Could you check a few things on this model? Use its own coordinates, in mm. Face numbers are marked on the shaded views. A direction names the side the tool comes from. Give positions to 0.01 mm unless a question says otherwise; leave off trailing zeros. Order: outer loops, then holes, each group sorted by start corner. A loop starts at its lowest first (then second) coordinate and runs counter-clockwise, first axis right, second up. Notation, with made-up numbers: (45, 33) -> (86, 33) arc R19 ccw to (86, 58) -> close; hole circle Ø11 at (14.25, 73.25). An arc over 180 degrees is marked (long way). Write each question's results on one line, items separated by ' | '.
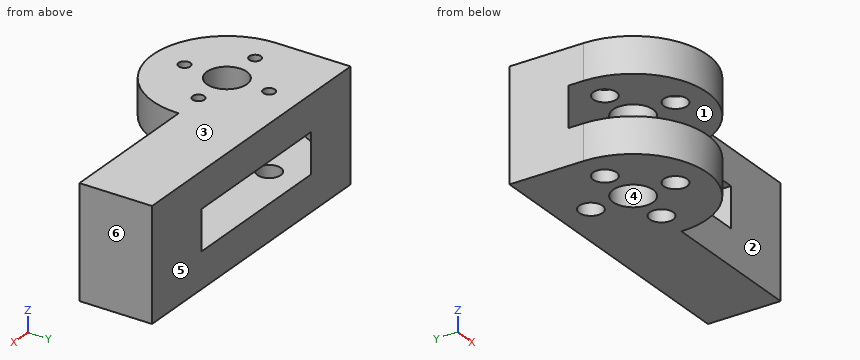
```python
from build123d import *

# Parameters (mm, degrees)
SKETCH1_R           = 3.429
BOSS_EXTRUDE1_DEPTH = 9.525
CUT_EXTRUDE1_START  = -9.525
CUT_EXTRUDE1_DEPTH  = 3.429
SKETCH4_R           = 1.004000024
CUT_EXTRUDE2_DEPTH  = 20.05
SKETCH5_R           = 2.000000064
CUT_EXTRUDE3_DEPTH  = 14.954


with BuildPart() as part:
    # Sketch1 → Boss-Extrude1 (new body, symmetric)
    with BuildSketch(Plane.XY):
        with BuildLine():
            Line((-12.7, 0), (-12.7, 12.7))
            Line((-12.7, 12.7), (38.1, 12.7))
            Line((38.1, 12.7), (38.1, 0.254))
            Line((38.1, 0.254), (12.697459746, 0.254))
            ThreePointArc((12.697459746, 0.254), (0.127006351, -12.699364921), (-12.7, 0))
        make_face()
        Circle(SKETCH1_R, mode=Mode.SUBTRACT)
    extrude(amount=BOSS_EXTRUDE1_DEPTH, both=True)

    # Sketch3 → Cut-Extrude1 (cut, symmetric)
    with BuildSketch(Plane.XY.offset(9.525).offset(CUT_EXTRUDE1_START)):
        with BuildLine():
            Line((25.4, 12.7), (25.4, 0.254))
            Line((25.4, 0.254), (12.951509565, 0.254))
            ThreePointArc((12.951509565, 0.254), (-9.069614104, -9.24922786), (0, 12.954))
            Line((0, 12.954), (0, 12.7))
            Line((0, 12.7), (25.4, 12.7))
        make_face()
    extrude(amount=CUT_EXTRUDE1_DEPTH, both=True, mode=Mode.SUBTRACT)

    # Sketch4 → Cut-Extrude2 (cut, through all)
    with BuildSketch(Plane.XY.offset(9.525)):
        with Locations((7.249999978, 0)):
            Circle(SKETCH4_R)
        with Locations((0, -7.249999978)):
            Circle(SKETCH4_R)
        with Locations((-7.249999978, 0)):
            Circle(SKETCH4_R)
        with Locations((0, 7.249999978)):
            Circle(SKETCH4_R)
    extrude(amount=-CUT_EXTRUDE2_DEPTH, mode=Mode.SUBTRACT)

    # Sketch5 → Cut-Extrude3 (cut)
    with BuildSketch(Plane(origin=(0, 0, -9.525), x_dir=(-1, 0, 0), z_dir=(0, 0, -1))):
        with Locations((7.249999978, 0)):
            Circle(SKETCH5_R)
        with Locations((0, -7.249999978)):
            Circle(SKETCH5_R)
        with Locations((-7.249999978, 0)):
            Circle(SKETCH5_R)
        with Locations((0, 7.249999978)):
            Circle(SKETCH5_R)
    extrude(amount=-CUT_EXTRUDE3_DEPTH, mode=Mode.SUBTRACT)


solid = part.part
```
Q1. Suppose I cut it at D-D on y = 7.25. Please give me the cut outline in (x, z) (3 decimals).
Here are the results:
outline: (-12.7, -9.525) -> (-2, -9.525) -> (-2, -3.429) -> (-10.735, -3.429) -> (-10.735, 3.429) -> (-2, 3.429) -> (-2, 5.429) -> (-1.004, 5.429) -> (-1.004, 9.525) -> (-12.7, 9.525) -> close; (1.004, 5.429) -> (2, 5.429) -> (2, 3.429) -> (25.4, 3.429) -> (25.4, -3.429) -> (2, -3.429) -> (2, -9.525) -> (38.1, -9.525) -> (38.1, 9.525) -> (1.004, 9.525) -> close
Q2. Suppose I cut it at A-A on x = 16. Please give me the cut outline in (y, z) (3 decimals).
Here are the results:
outline: (0.254, -9.525) -> (12.7, -9.525) -> (12.7, -3.429) -> (0.254, -3.429) -> close; (0.254, 3.429) -> (12.7, 3.429) -> (12.7, 9.525) -> (0.254, 9.525) -> close
Q3. For the marked faces 1, 2 and 3, which set-ups out of +Z, -Z, +X, -X, +Y, -Y let a thin tool reach every point of the face, with its end or its side?
Here are the results:
face 1: -Y | face 2: +Z, -Z, +X, -Y | face 3: +Z, +X, -X, +Y, -Y
Q4. I need wall thicknesses on line 1 along Y through (x, z) = (0, 3.9); line 2 along Z through (x, y) = (-8.5, 3.75) (3 decimals); line 3 along X through (y, z) = (7.25, 4.8). Which ranges of each line are inside material? Lowest first, please.
Here are the results:
line 1: y = -12.7 to -9.25, -5.25 to -3.43, 3.43 to 5.25, 9.25 to 12.7 | line 2: z = -9.525 to -3.429, 3.429 to 9.525 | line 3: x = -12.7 to -2, 2 to 38.1
Q5. Suppose I cut it at B-B on z = 2.25. Please give me the cut outline in (x, y).
Here are the results:
outline: (-12.7, 2.55) arc R12.95 cw to (-2.55, 12.7) -> (-12.7, 12.7) -> close; (25.4, 0.25) -> (38.1, 0.25) -> (38.1, 12.7) -> (25.4, 12.7) -> close
Q6. Thinking about a two-plate mould opening in Y: for the marked faces 4, 5 and 6, which applies, +Y half, -Y half, draft (parallel to the pull), parting line (faces both ways), or undercut?
Here are the results:
face 4: undercut | face 5: +Y half | face 6: draft
Q7. Suppose I cut it at C-C on x = 7. Please give me the cut outline in (y, z) (3 decimals).
Here are the results:
outline: (-10.597, -9.525) -> (-1.984, -9.525) -> (-1.984, -3.429) -> (-10.597, -3.429) -> close; (-10.597, 3.429) -> (-1.984, 3.429) -> (-1.984, 5.429) -> (-0.972, 5.429) -> (-0.972, 9.525) -> (-10.597, 9.525) -> close; (0.972, 5.429) -> (1.984, 5.429) -> (1.984, 3.429) -> (12.7, 3.429) -> (12.7, 9.525) -> (0.972, 9.525) -> close; (1.984, -9.525) -> (12.7, -9.525) -> (12.7, -3.429) -> (1.984, -3.429) -> close
Q8. I'm going to push flat-ended pins straight in: pin 1 Ø1.8 at (x, y) = (-7.25, 0) entering from +Z; pin 2 Ø3 at (x, y) = (-7.25, 0) entering from -Z. Where does each tip first touch, or does it pass through?
Here are the results:
pin 1: passes through | pin 2: stops at z = 5.43
